Input: part model. Units: mm. Frame: model coordinates. A direction names the side the tool comes from. Coordinates: 2 decimals unless noted, no trailing zeros. Order: outer loops, then holes, each group sorted by start corner. A loop starts at its lowest first (then second) coordinate and runs counter-clockwise, first axis right, second up. Notation, with made-up numbers: M 1,-15 L 8,-15 A25 cw 8,20 Z; hole C 25,-38.5 d10. An arc over 180 degrees is marked long. Answer in a Markdown table with one row per item.
from build123d import *

# Parameters (mm, degrees)
F0_R          = 70
F0_R_2        = 65
F1_DEPTH      = 2360
F2_W          = 200
F2_H          = 200
F2_R          = 11
F3_DEPTH      = 10
F4_W          = 30.1787997812
F4_H          = 10
F4_W_2        = 10
F4_H_2        = 30.1787997812
F5_DEPTH      = 150
F6_T1_DEPTH   = 269.311363913
F6_T3_DEPTH   = 269.311363913
F6_T8_DEPTH   = 269.311363913
F6_S9_R       = 70
F6_T10_DEPTH  = 139
F8_W          = 200
F8_H          = 200
F8_R          = 8.5
F9_DEPTH      = 10
F10_W         = 10
F10_H         = 30.1787997812
F10_W_2       = 30.1787997812
F10_H_2       = 10
F11_DEPTH     = 80
F12_T1_DEPTH  = 269.311363913
F12_T3_DEPTH  = 269.311363913
F12_T8_DEPTH  = 269.311363913
F12_S9_R      = 70
F12_T10_DEPTH = 139
F12_T14_DEPTH = 269.311363913
F12_S15_R     = 70
F12_T16_DEPTH = 139


# Not quite as in the source:
# - a fillet or chamfer that OpenCascade refuses, or shapes differently, is made with other operations: its cross-section is extruded or revolved along the edge and cut away or added


with BuildPart() as f1:
    # F0 (on Front) → F1 (new body)
    with BuildSketch(Plane.XZ):
        Circle(F0_R)
        Circle(F0_R_2, mode=Mode.SUBTRACT)
    extrude(amount=F1_DEPTH)

    # F2 (on Front) → F3 (join)
    with BuildSketch(Plane.XZ):
        Rectangle(F2_W, F2_H)
        with Locations((-75, -75)):
            Circle(F2_R, mode=Mode.SUBTRACT)
        with Locations((75, -75)):
            Circle(F2_R, mode=Mode.SUBTRACT)
        with Locations((-75, 75)):
            Circle(F2_R, mode=Mode.SUBTRACT)
        with Locations((75, 75)):
            Circle(F2_R, mode=Mode.SUBTRACT)
    extrude(amount=-F3_DEPTH)

    # F4 (on Front) → F5 (join)
    with BuildSketch(Plane.XZ):
        with Locations((-84.9106001094, 0)):
            Rectangle(F4_W, F4_H)
        with Locations((0, 84.9106001094)):
            Rectangle(F4_W_2, F4_H_2)
        with Locations((84.9106001094, 0)):
            Rectangle(F4_W, F4_H)
        with Locations((0, -84.9106001094)):
            Rectangle(F4_W_2, F4_H_2)
    extrude(amount=F5_DEPTH)

    # F6: chamfer of 50 x 20 on 4 edges, made by hand

    # F6_s2 → F6_t1 (cut)
    with BuildSketch(Plane.YZ.offset(-134.6556819565)):
        Polygon((-100, 100), (-150, 80), (-150, 100), align=None)
        Polygon((-100, -100), (-150, -80), (-150, -100), align=None)
    extrude(amount=F6_T1_DEPTH, mode=Mode.SUBTRACT)

    # F6_s4 → F6_t3 (cut)
    with BuildSketch(Plane.XY.offset(-134.6556819565)):
        Polygon((100, -100), (80, -150), (100, -150), align=None)
    extrude(amount=F6_T3_DEPTH, mode=Mode.SUBTRACT)


with BuildPart() as f6_tool6:
    # F6_s7 → F6_t8 (new body)
    with BuildSketch(Plane.XY.offset(134.6556819565)):
        Polygon((-100, -130), (-50, -150), (-100, -150), align=None)
    extrude(amount=-F6_T8_DEPTH)

    # F6_s9 → F6_t10 (cut, symmetric)
    with BuildSketch(Plane.XZ.offset(140)):
        Circle(F6_S9_R)
    extrude(amount=F6_T10_DEPTH, both=True, mode=Mode.SUBTRACT)


with BuildPart() as f1_1:
    add(f1.part)

    # F6_t5: cut F6_tool6
    add(f6_tool6.part, mode=Mode.SUBTRACT)

    # F8 (on offset) → F9 (join)
    with BuildSketch(Plane.XZ.offset(2360)):
        Rectangle(F8_W, F8_H)
        with Locations((-75, -75)):
            Circle(F8_R, mode=Mode.SUBTRACT)
        with Locations((75, -75)):
            Circle(F8_R, mode=Mode.SUBTRACT)
        with Locations((-75, 75)):
            Circle(F8_R, mode=Mode.SUBTRACT)
        with Locations((75, 75)):
            Circle(F8_R, mode=Mode.SUBTRACT)
    extrude(amount=F9_DEPTH)

    # F10 (on face) → F11 (join)
    with BuildSketch(Plane(origin=(0, -2360, 0), x_dir=(-1, 0, 0), z_dir=(0, 1, 0))):
        with Locations((0, 84.9106001094)):
            Rectangle(F10_W, F10_H)
        with Locations((84.9106001094, 0)):
            Rectangle(F10_W_2, F10_H_2)
        with Locations((0, -84.9106001094)):
            Rectangle(F10_W, F10_H)
        with Locations((-84.9106001094, 0)):
            Rectangle(F10_W_2, F10_H_2)
    extrude(amount=F11_DEPTH)

    # F12: chamfer of 20 x 50 on 4 edges, made by hand

    # F12_s2 → F12_t1 (cut)
    with BuildSketch(Plane.YZ.offset(-134.6556819565)):
        Polygon((-2330, 100), (-2280, 80), (-2280, 100), align=None)
    extrude(amount=F12_T1_DEPTH, mode=Mode.SUBTRACT)

    # F12_s4 → F12_t3 (cut)
    with BuildSketch(Plane.XY.offset(-134.6556819565)):
        Polygon((100, -2330), (80, -2280), (100, -2280), align=None)
    extrude(amount=F12_T3_DEPTH, mode=Mode.SUBTRACT)


with BuildPart() as f12_tool6:
    # F12_s7 → F12_t8 (new body)
    with BuildSketch(Plane.XY.offset(-134.6556819565)):
        Polygon((-100, -2300), (-50, -2280), (-100, -2280), align=None)
    extrude(amount=F12_T8_DEPTH)

    # F12_s9 → F12_t10 (cut, symmetric)
    with BuildSketch(Plane.XZ.offset(2290)):
        Circle(F12_S9_R)
    extrude(amount=F12_T10_DEPTH, both=True, mode=Mode.SUBTRACT)


with BuildPart() as f1_2:
    add(f1_1.part)

    # F12_t5: cut F12_tool6
    add(f12_tool6.part, mode=Mode.SUBTRACT)


with BuildPart() as f12_tool12:
    # F12_s13 → F12_t14 (new body)
    with BuildSketch(Plane.YZ.offset(134.6556819565)):
        Polygon((-2300, -100), (-2280, -50), (-2280, -100), align=None)
    extrude(amount=-F12_T14_DEPTH)

    # F12_s15 → F12_t16 (cut, symmetric)
    with BuildSketch(Plane.XZ.offset(2290)):
        Circle(F12_S15_R)
    extrude(amount=F12_T16_DEPTH, both=True, mode=Mode.SUBTRACT)


with BuildPart() as f1_3:
    add(f1_2.part)

    # F12_t11: cut F12_tool12
    add(f12_tool12.part, mode=Mode.SUBTRACT)


solid = f1_3.part
1) Cut plane B-B, the plane x = -30. Output: boundary loops of the cut face in (y, z).
Resolved:
| item | result |
|---|---|
| outline | M -2370,-100 L -2360,-100 L -2360,-63.25 L 0,-63.25 L 0,-100 L 10,-100 L 10,100 L 0,100 L 0,63.25 L -2360,63.25 L -2360,100 L -2370,100 Z; hole M -2360,-57.66 L 0,-57.66 L 0,57.66 L -2360,57.66 Z |
2) Cut plane A-A, the plane y = -560. Output: boundary loops of the cut face in (x, z).
Resolved:
| item | result |
|---|---|
| outline | C 0,0 d140; hole C 0,0 d130 |
3) Material intervals for probe 1 along Z at (x, y) = (-75, 5); probe 2 along Y at (x, z) = (28, 37); probe 3 along Z at (x, y) = (16, -690.5), sorted ascending.
Resolved:
| item | result |
|---|---|
| probe 1 | z = -100 to -86, -64 to 64, 86 to 100 |
| probe 2 | y = -2370 to -2360, 0 to 10 |
| probe 3 | z = -68.15 to -63, 63 to 68.15 |
4) Reachability of faces 4 (the face through (-64, -2360, 64)), 5 (the face through (62, 0, 64)), 6 (the face through (-64, -2360, -62)), 7 (the face through (0, -13, 100)), 8 (the face through (-1, 0, 1)) from +Z, -Z, +X, -X, +Y, -Y: full face, straight path, thin tool, end or side. Return the list, or none.
Resolved:
| item | result |
|---|---|
| face 4 | +Z, -X |
| face 5 | +Z, +X |
| face 6 | -Z, -X |
| face 7 | +Z, +X, -X, +Y, -Y |
| face 8 | none |
5) Mould query, pull axis Z, two halves, no side actions, for faces 1 (the face through (62, -1163.48, 19.52)), 2 (the face through (64.662, -1163.48, -26.81)), 3 (the face through (62, 0, -62)). Classes: +Z half, -Z half, draft (parallel to the pull), parting line (faces both ways), or undercut.
Resolved:
| item | result |
|---|---|
| face 1 | undercut |
| face 2 | parting line |
| face 3 | draft |
6) Contact query for flat-ended pins moving along their axis: pin 1 (8 mm diameter, centred on y = -986, z = -75.5, fed in from +X); pin 2 (8 mm diameter, centred on y = -879.5, z = -33.5, fed in from +X); pin 3 (3 mm diameter, centred on x = 1.5, y = -627.5, fed in from +Z); pin 4 (15 mm diameter, centred on x = 87.5, y = -2324, fed in from +Z). Output: stop coordinate, or through.
Resolved:
| item | result |
|---|---|
| pin 1 | passes through |
| pin 2 | stops at x = 63.48 |
| pin 3 | stops at z = 70 |
| pin 4 | stops at z = 5 |
